Check sheet for the modelled part. Datum: model origin and axes. Units: mm. Round coordinates to 2 decimals unless told otherwise and drop trailing zeros. Loops run counter-clockwise (first coordinate to the right, second up) from the corner with the lowest first, then second, coordinate; pieces in that order, holes last. Notation, with made-up numbers: M 34,15 L 42,15 A35 ccw 42,50 Z; hole C -38,27.5 d2. An arc over 180 degrees is marked long. One line per question, with ' | ' between items. Start each with the question number.
(1) Section check B-B (y = 25.25). Record the boundary of the cut face in (x, z), and give its area (3 significant figures).
(2) Section check A-A (x = 83). Record the boundary of the cut face in (y, z), and give its area (3 significant figures).
(3) Draft check along X on faces 1 (the face through (97.3, 25.8, 2.5)), 2 (the face through (91, 26, 5)), 3 (the face through (77, 26, 2)). Enter one of: +X half, -X half, draft (parallel to the pull), parting line (faces both ways), or undercut.
(4) Thickness scan on probe 1 along X at (y, z) = (25.75, 1.9); probe 2 along X at (y, z) = (27.25, 2.05); probe 3 along Y at (x, z) = (83, 1.75). Record the ranges inside material, lowest first. Write a range as [from, to].
(5) Section check D-D (y = 27.25). Record the boundary of the cut face in (x, z).
(6) Go/stop test with a flat-tipped pin: P1, Ø1, axis at x = 91, y = 21.5, coming from the -Z side. Record where the tip stops, or that it passes through.
(7) Section check C-C (z = 2.1). Record the boundary of the cut face in (x, y).
Solid Edge part; units mm, degrees
sketch "Sketch1" plane through (0, 0, 0) normal (0, 0, 1) x (1, 0, 0)
  circle A0 centre (99, 25.8394) radius 1.7
  line L0 (77, 19.8394) -> (105, 19.8394)
  line L1 (105, 19.8394) -> (105, 31.8394)
  line L2 (105, 31.8394) -> (77, 31.8394)
  line L3 (77, 31.8394) -> (77, 19.8394)
  circle A1 centre (83, 25.8394) radius 1.7
  dimension "D1" = 77
  dimension "D2" = 105
extrude "Protrusion1" add sketch "Sketch1" along normal blind 5
properties material "ABS Plastic, high impact"
The answers:
1) outline: M 77,0 L 81.41,0 L 81.41,5 L 77,5 Z; M 84.59,0 L 97.41,0 L 97.41,5 L 84.59,5 Z; M 100.59,0 L 105,0 L 105,5 L 100.59,5 Z | area: 108 mm²
2) outline: M 19.84,0 L 24.14,0 L 24.14,5 L 19.84,5 Z; M 27.54,0 L 31.84,0 L 31.84,5 L 27.54,5 Z | area: 43.0 mm²
3) face 1: undercut | face 2: draft | face 3: -X half
4) probe 1: [77, 81.3], [84.7, 97.3], [100.7, 105] | probe 2: [77, 82.05], [83.95, 98.05], [99.95, 105] | probe 3: [19.84, 24.14], [27.54, 31.84]
5) outline: M 77,0 L 82.05,0 L 82.05,5 L 77,5 Z; M 83.95,0 L 98.05,0 L 98.05,5 L 83.95,5 Z; M 99.95,0 L 105,0 L 105,5 L 99.95,5 Z
6) P1: z = 0
7) outline: M 77,19.84 L 105,19.84 L 105,31.84 L 77,31.84 Z; hole C 83,25.84 d3.4; hole C 99,25.84 d3.4
